from build123d import *

# Parameters (mm, degrees)
F0_R     = 16.5
F0_W     = 12.3
F0_H     = 12.2936
F1_DEPTH = 25.4
F2_R     = 16.5
F3_DEPTH = 50.8


with BuildPart() as f1:
    # F0 (on Front) → F1 (new body)
    with BuildSketch(Plane.XZ):
        Circle(F0_R)
        Rectangle(F0_W, F0_H, mode=Mode.SUBTRACT)
    extrude(amount=F1_DEPTH)

    # F2 (on face) → F3 (join)
    with BuildSketch(Plane.XZ.offset(25.4)):
        Circle(F2_R)
    extrude(amount=F3_DEPTH)


solid = f1.part
Geometry check sheet. Reference: the model listing, model coordinates, mm. A direction names the side the tool comes from. Round coordinates to 2 decimals unless told otherwise and drop trailing zeros. Order: outer loops, then holes, each group sorted by start corner. A loop starts at its lowest first (then second) coordinate and runs counter-clockwise, first axis right, second up. Notation, with made-up numbers: M 6.5,60.25 L 42.5,60.25 A14 cw 42.5,76.25 Z; hole C 44,50.25 d1. An arc over 180 degrees is marked long. Answer in a Markdown table with one row per item. Add a question column.
Item 1: Sectioned sample at C-C, the plane x = 0. Enter the section's corners in (y, z).
Item 2: Depth check by flat-ended pin: pin 1 Ø4 at (y, z) = (-64, 5.5) entering from +X; pin 2 Ø2 at (x, y) = (-10.5, -57) entering from +Z; pin 3 Ø8 at (y, z) = (-60.5, 6.5) entering from -X. Enter the tip coordinate at first touch or a pass-through.
Item 3: Set-up check for faces 1 (the face through (0, -13, -6.147)), 2 (the face through (0, -76.2, 0)): record each of +Z, -Z, +X, -X, +Y, -Y from which the full face is reachable in a straight line by a thin tool's end or side.
Item 4: Material ranges on L1, parallel to Y at x = -2.5, z = -2.5; L2, parallel to Z at x = -5, y = -8.5; L3, parallel to X at y = -24.5, z = 1.5, recorded low to high. Write a range as [from, to].
Item 5: Draft check along Z on faces 3 (the face through (15.24, -37.57, -6.32)), 4 (the face through (6.15, -13, 0)), 5 (the face through (0, 0, -7)). Enter one of: released by +Z, released by -Z, zero draft, split by the parting line, or undercut.
Item 6: Sectioned sample at A-A, the plane y = -7.5. Enter the section's corners in (x, z).
Item 7: Sectioned sample at D-D, the plane y = -49. Enter the section's corners in (x, z), plus the area to 3 significant figures.
Item 8: Sectioned sample at B-B, the plane z = 0. Enter the section's corners in (x, y), plus the area to 3 significant figures.
Filled in:
| question | item | result |
|---|---|---|
| 1 | outline | M -76.2,-16.5 L 0,-16.5 L 0,-6.15 L -25.4,-6.15 L -25.4,6.15 L 0,6.15 L 0,16.5 L -76.2,16.5 Z |
| 2 | pin 1 | stops at x = 16.12 |
| 2 | pin 2 | stops at z = 13.49 |
| 2 | pin 3 | stops at x = -16.31 |
| 3 | face 1 | +Y |
| 3 | face 2 | +Z, -Z, +X, -X, -Y |
| 4 | L1 | y = [-76.2, -25.4] |
| 4 | L2 | z = [-15.72, -6.15], [6.15, 15.72] |
| 4 | L3 | x = [-16.43, -6.15], [6.15, 16.43] |
| 5 | face 3 | split by the parting line |
| 5 | face 4 | undercut |
| 5 | face 5 | zero draft |
| 6 | outline | C 0,0 d33; hole M -6.15,-6.15 L 6.15,-6.15 L 6.15,6.15 L -6.15,6.15 Z |
| 7 | outline | C 0,0 d33 |
| 7 | area | 855 mm² |
| 8 | outline | M -16.5,-76.2 L 16.5,-76.2 L 16.5,0 L 6.15,0 L 6.15,-25.4 L -6.15,-25.4 L -6.15,0 L -16.5,0 Z |
| 8 | area | 2,200 mm² |
